from build123d import *

# Parameters (mm, degrees)
F1_DEPTH = 5
F3_DEPTH = 25
F4_R     = 1
F5_DEPTH = 5


with BuildPart() as f1:
    # F0 (on Front) → F1 (new body)
    with BuildSketch(Plane.XZ):
        Polygon((-54.360465, 2), (-54.360465, 0), (-53.141715, 0), (-53.860465, 2), align=None)
        Polygon((-53.141715, 0), (-54.360465, 0), (-54.360465, -5), (55.639535, -5), (55.639535, 0), (54.420785, 0), (53.920785, 0), (53.420785, 0), (50.983285, 0), (50.483285, 0), (49.983285, 0), (47.545785, 0), (47.045785, 0), (46.545785, 0), (44.108285, 0), (43.608285, 0), (43.108285, 0), (40.670785, 0), (40.170785, 0), (39.670785, 0), (37.233285, 0), (36.733285, 0), (36.233285, 0), (33.795785, 0), (33.295785, 0), (32.795785, 0), (30.358285, 0), (29.858285, 0), (29.358285, 0), (26.920785, 0), (26.420785, 0), (25.920785, 0), (23.483285, 0), (22.983285, 0), (22.483285, 0), (20.045785, 0), (19.545785, 0), (19.045785, 0), (16.608285, 0), (16.108285, 0), (15.608285, 0), (13.170785, 0), (12.670785, 0), (12.170785, 0), (9.733285, 0), (9.233285, 0), (8.733285, 0), (6.295785, 0), (5.795785, 0), (5.295785, 0), (2.858285, 0), (2.358285, 0), (1.858285, 0), (-0.579215, 0), (-1.079215, 0), (-1.579215, 0), (-4.016715, 0), (-4.516715, 0), (-5.016715, 0), (-7.454215, 0), (-7.954215, 0), (-8.454215, 0), (-10.891715, 0), (-11.391715, 0), (-11.891715, 0), (-14.329215, 0), (-14.829215, 0), (-15.329215, 0), (-17.766715, 0), (-18.266715, 0), (-18.766715, 0), (-21.204215, 0), (-21.704215, 0), (-22.204215, 0), (-24.641715, 0), (-25.141715, 0), (-25.641715, 0), (-28.079215, 0), (-28.579215, 0), (-29.079215, 0), (-31.516715, 0), (-32.016715, 0), (-32.516715, 0), (-34.954215, 0), (-35.454215, 0), (-35.954215, 0), (-38.391715, 0), (-38.891715, 0), (-39.391715, 0), (-41.829215, 0), (-42.329215, 0), (-42.829215, 0), (-45.266715, 0), (-45.766715, 0), (-46.266715, 0), (-48.704215, 0), (-49.204215, 0), (-49.704215, 0), (-52.141715, 0), (-52.641715, 0), align=None)
        Polygon((-51.422965, 2), (-52.141715, 0), (-49.704215, 0), (-50.422965, 2), (-50.922965, 2), align=None)
        Polygon((54.420785, 0), (55.639535, 0), (55.639535, 2), (55.139535, 2), align=None)
        Polygon((-47.985465, 2), (-48.704215, 0), (-46.266715, 0), (-46.985465, 2), (-47.485465, 2), align=None)
        Polygon((50.983285, 0), (53.420785, 0), (52.702035, 2), (52.202035, 2), (51.702035, 2), align=None)
        Polygon((-44.547965, 2), (-45.266715, 0), (-42.829215, 0), (-43.547965, 2), (-44.047965, 2), align=None)
        Polygon((47.545785, 0), (49.983285, 0), (49.264535, 2), (48.764535, 2), (48.264535, 2), align=None)
        Polygon((-41.110465, 2), (-41.829215, 0), (-39.391715, 0), (-40.110465, 2), (-40.610465, 2), align=None)
        Polygon((44.108285, 0), (46.545785, 0), (45.827035, 2), (45.327035, 2), (44.827035, 2), align=None)
        Polygon((-37.672965, 2), (-38.391715, 0), (-35.954215, 0), (-36.672965, 2), (-37.172965, 2), align=None)
        Polygon((40.670785, 0), (43.108285, 0), (42.389535, 2), (41.889535, 2), (41.389535, 2), align=None)
        Polygon((-34.235465, 2), (-34.954215, 0), (-32.516715, 0), (-33.235465, 2), (-33.735465, 2), align=None)
        Polygon((37.233285, 0), (39.670785, 0), (38.952035, 2), (38.452035, 2), (37.952035, 2), align=None)
        Polygon((-30.797965, 2), (-31.516715, 0), (-29.079215, 0), (-29.797965, 2), (-30.297965, 2), align=None)
        Polygon((33.795785, 0), (36.233285, 0), (35.514535, 2), (35.014535, 2), (34.514535, 2), align=None)
        Polygon((-27.360465, 2), (-28.079215, 0), (-25.641715, 0), (-26.360465, 2), (-26.860465, 2), align=None)
        Polygon((30.358285, 0), (32.795785, 0), (32.077035, 2), (31.577035, 2), (31.077035, 2), align=None)
        Polygon((-23.922965, 2), (-24.641715, 0), (-22.204215, 0), (-22.922965, 2), (-23.422965, 2), align=None)
        Polygon((26.920785, 0), (29.358285, 0), (28.639535, 2), (28.139535, 2), (27.639535, 2), align=None)
        Polygon((-20.485465, 2), (-21.204215, 0), (-18.766715, 0), (-19.485465, 2), (-19.985465, 2), align=None)
        Polygon((23.483285, 0), (25.920785, 0), (25.202035, 2), (24.702035, 2), (24.202035, 2), align=None)
        Polygon((-17.047965, 2), (-17.766715, 0), (-15.329215, 0), (-16.047965, 2), (-16.547965, 2), align=None)
        Polygon((20.045785, 0), (22.483285, 0), (21.764535, 2), (21.264535, 2), (20.764535, 2), align=None)
        Polygon((-13.610465, 2), (-14.329215, 0), (-11.891715, 0), (-12.610465, 2), (-13.110465, 2), align=None)
        Polygon((16.608285, 0), (19.045785, 0), (18.327035, 2), (17.827035, 2), (17.327035, 2), align=None)
        Polygon((-10.172965, 2), (-10.891715, 0), (-8.454215, 0), (-9.172965, 2), (-9.672965, 2), align=None)
        Polygon((13.170785, 0), (15.608285, 0), (14.889535, 2), (14.389535, 2), (13.889535, 2), align=None)
        Polygon((-6.735465, 2), (-7.454215, 0), (-5.016715, 0), (-5.735465, 2), (-6.235465, 2), align=None)
        Polygon((9.733285, 0), (12.170785, 0), (11.452035, 2), (10.952035, 2), (10.452035, 2), align=None)
        Polygon((-3.297965, 2), (-4.016715, 0), (-1.579215, 0), (-2.297965, 2), (-2.797965, 2), align=None)
        Polygon((6.295785, 0), (8.733285, 0), (8.014535, 2), (7.514535, 2), (7.014535, 2), align=None)
        Polygon((0.139535, 2), (-0.579215, 0), (1.858285, 0), (1.139535, 2), (0.639535, 2), align=None)
        Polygon((2.858285, 0), (5.295785, 0), (4.577035, 2), (4.077035, 2), (3.577035, 2), align=None)
    extrude(amount=F1_DEPTH)

    # F2 (on face) → F3 (cut)
    with BuildSketch(Plane.XZ.offset(5)):
        Polygon((40.639535, 9.693892), (40.639535, -5), (40.639535, -8.513346), (59.679061, -8.513346), (59.679061, 9.693892), align=None)
    extrude(amount=-F3_DEPTH, mode=Mode.SUBTRACT)

    # F4 (on face) → F5 (join, through all)
    with BuildSketch(Plane.XZ.offset(5)):
        with BuildLine():
            Line((40.639535, 0), (40.639535, -5))
            Line((40.639535, -5), (42.509039, -4.065248))
            ThreePointArc((42.509039, -4.065248), (43.215055, -3.420029), (43.476416, -2.5))
            ThreePointArc((43.476416, -2.5), (43.215055, -1.579971), (42.509039, -0.934752))
            Line((42.509039, -0.934752), (40.639535, 0))
        make_face()
        with Locations((41.726416, -2.5)):
            Circle(F4_R, mode=Mode.SUBTRACT)
    extrude(amount=-F5_DEPTH)


solid = f1.part
Source: CAD feature listing. Evaluate the final solid. Frame: model axes, mm. Give positions to 0.01 mm unless a question says otherwise; leave off trailing zeros. Return JSON: item names as keys, results as strings. Group by question number.
1) Pull-direction query (X, two-part tool) for faces 1 (the face through (29, -2, 1)), 2 (the face through (-8, -2, -5)), 3 (the face through (-54.36, -2, -1)); classes: pulls with the +X half, pulls with the -X half, needs draft (parallel to the pull), parting line crosses it, or undercut.
2) Pin query (flat end, axial travel): P1, Ø0.5, axis at x = -8, y = -1.5, coming from the +Z side; P2, Ø3, axis at y = -3, z = -1.5, coming from the +X side; P3, Ø2, axis at y = -1, z = -0.5, coming from the +X side. Return the tip coordinate at first contact, or that it passes through.
3) Material intervals for line 1 along Z through (x, y) = (12.5, -2.4); line 2 along X through (y, z) = (-1.35, -1.75), sorted ascending. Write a range as [from, to].
Recorded:
{
 "1": {"face 1": "undercut", "face 2": "needs draft", "face 3": "pulls with the -X half"},
 "2": {"P1": "stops at z = 0", "P2": "stops at x = 43.48", "P3": "stops at x = 43.16"},
 "3": {"line 1": "z = [-5, 0]", "line 2": "x = [-54.36, 41.06], [42.39, 43.31]"}
}
